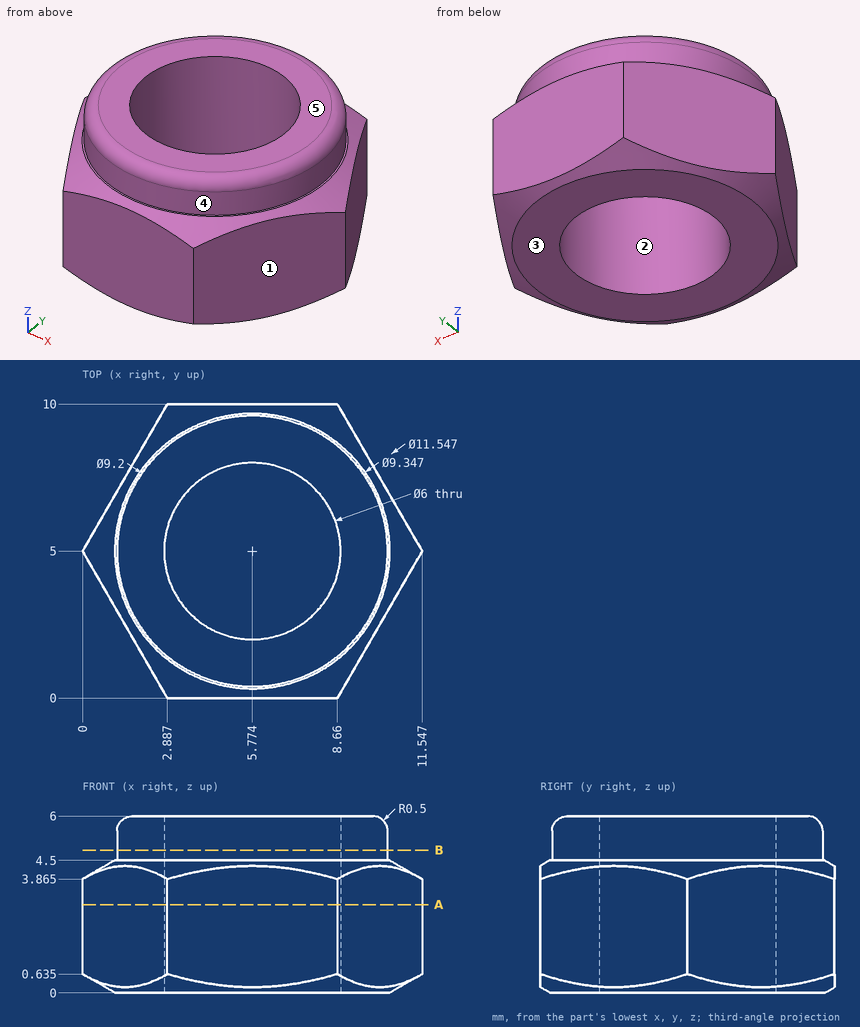
Study the drawing (mm; zero at the part's minimum x, y, z) and answer. A direction names the side the tool comes from. Coordinates: 2 decimals unless noted, no trailing zeros. Order: outer loops, then holes, each group sorted by start corner. A loop starts at its lowest first (then second) coordinate and runs counter-clockwise, first axis right, second up. Notation, with made-up numbers: (-2, 43.25) -> (51, 43.25) arc R25 cw to (51, 56.25) -> close; hole circle Ø3 at (-18.75, 21.5). An arc over 180 degrees is marked (long way). Answer in a Markdown table with one row per item. Add a question column.
Item 1: Find the intervals of material crossed by L1, parallel to X at y = 7.5, z = 2.6 (1 decimal); L2, parallel to Y at x = 5.25, z = 5.6 (1 decimal); L3, parallel to X at y = 7, z = 1 (1 decimal), in increasing order. Write a range as from..to.
Item 2: Determine the mould class of the marked faces 1, 2 and 3 for opening direction Y: +Y half, -Y half, draft (parallel to the pull), parting line (faces both ways), or undercut.
Item 3: Find section B-B (z = 4.85). Write down the section's boundary in (x, y), then the cut area to 3 significant figures.
Item 4: Which of the six approach directions +Z, -Z, +X, -X, +Y, -Y give full straight-line access (tool end or side, diameter ignored) to the marked faces 4 and 5?
Item 5: Find section A-A (z = 3). Write down the section's boundary in (x, y).
Item 6: Each of these flat-tipped pins is pushed along its axis until it touches: P1, Ø1, axis at x = 10, y = 1.5, coming from the -Z side; P2, Ø1, axis at x = 1.5, z = 4, coming from the -Y side (1 decimal). Where does it stop, or does it pass through?
Result set:
| question | item | result |
|---|---|---|
| 1 | L1 | x = 1.4..4.1, 7.4..10.1 |
| 1 | L2 | y = 0.4..2, 8..9.6 |
| 1 | L3 | x = 1.2..3.5, 8..10.4 |
| 2 | face 1 | -Y half |
| 2 | face 2 | undercut |
| 2 | face 3 | draft |
| 3 | outline | circle Ø9.2 at (5.77, 5); hole circle Ø6 at (5.77, 5) |
| 3 | area | 38.2 mm² |
| 4 | face 4 | +Z |
| 4 | face 5 | +Z, +X, -X, +Y, -Y |
| 5 | outline | (0, 5) -> (2.89, 0) -> (8.66, 0) -> (11.55, 5) -> (8.66, 10) -> (2.89, 10) -> close; hole circle Ø6 at (5.77, 5) |
| 6 | P1 | stops at z = 0.18 |
| 6 | P2 | stops at y = 1.5 |
